```python
from build123d import *

# Parameters (mm, degrees)
BOSS_EXTRU_1_DEPTH = 2
CONG_1_R           = 4
CONG_2_R           = 1


with BuildPart() as part:
    # Esquisse1 → Boss.-Extru.1 (new body)
    with BuildSketch(Plane.XY):
        Polygon((0, 5.75), (2.675426481, 5.75), (2.675426481, 4.75), (7.775426481, 4.75), (7.775426481, 4.95), (10.350852961, 4.75), (10.350852961, -4.75), (7.775426481, -4.95), (7.775426481, -4.75), (2.675426481, -4.75), (2.675426481, -5.75), (0, -5.75), align=None)
        Polygon((2, 0), (3.58771324, -2.75), (6.763139721, -2.75), (8.350852961, 0), (6.763139721, 2.75), (3.58771324, 2.75), align=None, mode=Mode.SUBTRACT)
    extrude(amount=BOSS_EXTRU_1_DEPTH)

    # Congé1
    # the kernel refuses this fillet: 4 mm, written as the material it takes off along each edge
    with BuildSketch(Plane(origin=(0, -5.75, -9.435804481), x_dir=(1, 0, 0), z_dir=(0, 0, 1))) as cong_1_piece_1:
        with BuildLine():
            CenterArc((4, 3.774321792), CONG_1_R, 180, 70.661811314)
            Line((0, 3.774321792), (-0.08, 3.774321792))
            Line((-0.08, 3.774321792), (-0.08, 0))
            Line((-0.08, 0), (0, -0.08))
            ThreePointArc((0, -0.08), (1.33771324, -0.08), (2.64893501, -0.075486436))
            Line((2.64893501, -0.075486436), (2.675426481, 0))
        make_face()
    extrude(amount=20.871608961, mode=Mode.SUBTRACT)
    with BuildSketch(Plane(origin=(0, 5.75, -9.435804481), x_dir=(1, 0, 0), z_dir=(0, 0, 1))) as cong_1_piece_2:
        with BuildLine():
            CenterArc((4, -3.774321792), CONG_1_R, 109.338188686, 70.661811314)
            Line((0, -3.774321792), (-0.08, -3.774321792))
            Line((-0.08, -3.774321792), (-0.08, 0))
            Line((-0.08, 0), (0, 0.08))
            ThreePointArc((0, 0.08), (1.33771324, 0.08), (2.64893501, 0.075486436))
            Line((2.64893501, 0.075486436), (2.675426481, 0))
        make_face()
    extrude(amount=20.871608961, mode=Mode.SUBTRACT)

    # Congé2
    cong_2_edges = [part.edges().sort_by_distance(p)[0] for p in [
        (10.350852961, 4.75, 1),
        (10.350852961, -4.75, 1),
    ]]
    fillet(cong_2_edges, radius=CONG_2_R)


solid = part.part
```
For this review, take the finished solid that the model builds, in its own axes (mm). A direction names the side the tool comes from. Coordinates: 2 decimals unless noted, no trailing zeros. Write each loop counter-clockwise with the first axis right and the second up, starting at its lowest first coordinate (ties: lowest second). Pieces come first, ordered by that corner, then holes. Notation, with made-up numbers: (47, 14.25) - (81, 14.25) arc R22 cw to (81, 38.25) - close; hole circle Ø1 at (30.25, 29.25). An arc over 180 degrees is marked (long way). Answer in a Markdown table with one row per item. Add a question column.
Q1. Tool access review of faces 5 (the flat face through (7.55, -1.39, 0.99)), 6 (the flat face through (1.8, 0.1, 2)), 7 (the flat face through (2.675, 5, 1)), 8 (the flat face through (2.675, -5, 1)), 9 (the cylindrical face through (0.76, 4.32, 0.99)): name each direction out of +Z, -Z, +X, -X, +Y, -Y from which nothing blocks a thin tool from reaching the whole face with its end or side.
Q2. Draft analysis for pull direction Y (two halves, no side actions). For faces 1 (the flat face through (5, -2.75, 1)), 2 (the flat face through (0, 0, 1)), 3 (the flat face through (2.783, -1.356, 0.986)), 4 (the cylindrical face through (10.09, 4.5, 1.01)), state which applies: +Y half, -Y half, draft (parallel to the pull), parting line (faces both ways), or undercut.
Q3. We need section D-D, the plane x = 1.25. State the section outline as (y, z) points, and give its area (3 significant figures).
Q4. For probe 1 along Y at (x, z) = (6.25, 1.65); probe 2 along X at (y, z) = (1.75, 0.75); probe 3 along Y at (x, z) = (3.5, 1.3), list the stretches that pass through material, from the lowest coordinate up.
Q5. We need section A-A, the plane x = 5.5. State the section outline as (y, z) points.
Q6. We need section C-C, the plane z = 1.85. State the section outline as (x, y) points, and give its area (3 significant figures).
Q7. For P1, Ø0.8, axis at y = -5, z = 0.5, coming from the +X side; P2, Ø0.5, axis at y = 5.5, z = 1, coming from the +X side; P3, Ø0.6, axis at x = 4.5, z = 1, coming from the -Y side, all flat-tipped, find the tip position at first contact; note any pin that passes through.
Q8. We need section B-B, the plane y = -0.75. State the section outline as (x, z) points, and give its area (3 significant figures).
Answer list:
| question | item | result |
|---|---|---|
| 1 | face 5 | +Z, -Z |
| 1 | face 6 | +Z, +X, -X, +Y, -Y |
| 1 | face 7 | +Z, -Z, +Y |
| 1 | face 8 | +Z, -Z, -Y |
| 1 | face 9 | +Z, -Z, -X, +Y |
| 2 | face 1 | undercut |
| 2 | face 2 | draft |
| 2 | face 3 | undercut |
| 2 | face 4 | +Y half |
| 3 | outline | (-4.88, 0) - (4.88, 0) - (4.88, 2) - (-4.88, 2) - close |
| 3 | area | 19.5 mm2 |
| 4 | probe 1 | y = -4.75 to -2.75, 2.75 to 4.75 |
| 4 | probe 2 | x = 0 to 3.01, 7.34 to 10.35 |
| 4 | probe 3 | y = -4.75 to -2.6, 2.6 to 4.75 |
| 5 | outline | (-4.75, 0) - (-2.75, 0) - (-2.75, 2) - (-4.75, 2) - close; (2.75, 0) - (4.75, 0) - (4.75, 2) - (2.75, 2) - close |
| 6 | outline | (0, -1.98) arc R4 ccw to (2.68, -5.75) - (2.68, -4.75) - (7.78, -4.75) - (7.78, -4.95) - (9.43, -4.82) arc R1 ccw to (10.35, -3.82) - (10.35, 3.82) arc R1 ccw to (9.43, 4.82) - (7.78, 4.95) - (7.78, 4.75) - (2.68, 4.75) - (2.68, 5.75) arc R4 ccw to (0, 1.98) - close; hole (2, 0) - (3.59, -2.75) - (6.76, -2.75) - (8.35, 0) - (6.76, 2.75) - (3.59, 2.75) - close |
| 6 | area | 72.2 mm2 |
| 7 | P1 | stops at x = 9.98 |
| 7 | P2 | stops at x = 2.68 |
| 7 | P3 | stops at y = -4.75 |
| 8 | outline | (0, 0) - (2.43, 0) - (2.43, 2) - (0, 2) - close; (7.92, 0) - (10.35, 0) - (10.35, 2) - (7.92, 2) - close |
| 8 | area | 9.73 mm2 |
